Geometry: final body of the model. Coordinates: model frame, mm. A direction names the side the tool comes from. Round coordinates to 2 decimals unless told otherwise and drop trailing zeros. Loops run counter-clockwise (first coordinate to the right, second up) from the corner with the lowest first, then second, coordinate; pieces in that order, holes last. Notation, with made-up numbers: (-10.75, -11.75) - (47.25, -11.75) arc R25 cw to (47.25, 23.25) - close; hole circle Ø2 at (53.5, -14.5). An arc over 180 degrees is marked (long way). Answer as a JSON object with one key per item and string values. Group by question number.
Item 1: Section A-A (z = 0.25). Return the cut outline in (x, y).
Item 2: First-contact query: pin 1 (1 mm diameter, centred on x = -0.5, y = 4.5, fed in from -Z); pin 2 (1.5 mm diameter, centred on x = 1.5, y = 8.5, fed in from +Z); pin 3 (5 mm diameter, centred on y = 8, z = 1, fed in from +X). Flat tips, straight axial feed; report the tip coordinate or a pass-through.
Item 3: Reachability of faces 4 (the face through (0, 12, -3)), 5 (the face through (6.554, 6, 0)), 6 (the face through (0.103, 6.085, -5.885)), 7 (the face through (-2.1, 10.8, 5.8)), 8 (the face through (0, 12, 3)) from +Z, -Z, +X, -X, +Y, -Y: full face, straight path, thin tool, end or side. Return the list, or none.
Item 4: Line query: line 1 (Y direction, x = 6.5, z = 4.75); line 2 (X direction, y = -0.5, z = -4.75); line 3 (X direction, y = 3, z = -0.75). Output: solid intervals per line, ascending.
Item 5: Draft query along Y for faces 1 (the face through (-7.1, 12, 0)), 2 (the face through (0, 0, 0)), 3 (the face through (-2.1, 1.5, 5.8)). Return one class per face: released by +Y, released by -Y, zero draft, split by the parting line, or undercut.
Item 6: Section C-C (y = 7.25). Return the cut outline in (x, z), plus the area to 3 significant figures.
Item 7: Section B-B (x = -3.5). Return the cut outline in (y, z).
Item 8: Section D-D (x = -6). Return the cut outline in (y, z).
```python
from build123d import *

# Parameters (mm, degrees)
SKETCH_1_W           = 14.2
SKETCH_1_H           = 12.2
EXTRUDE_1_DEPTH      = 12.8
SKETCH_2_OUTSIDE_W   = 20.736
SKETCH_2_OUTSIDE_H   = 18.736
SKETCH_2_OUTSIDE_W_2 = 19.736348523
SKETCH_2_OUTSIDE_H_2 = 6
CUT_EXTRUDE_1_DEPTH  = 1.5
SKETCH_3_OUTSIDE_W   = 20.736
SKETCH_3_OUTSIDE_H   = 18.736
CUT_EXTRUDE_2_DEPTH  = 9.3
SKETCH_4_R           = 0.375
EXTRUDE_2_DEPTH      = 4.5


with BuildPart() as part:
    # 草图1 → 凸台-拉伸1 (new body)
    with BuildSketch(Plane(origin=(0, 0, 0), x_dir=(1, 0, 0), z_dir=(0, 1, 0))):
        Rectangle(SKETCH_1_W, SKETCH_1_H)
    extrude(amount=EXTRUDE_1_DEPTH)

    # 草图2 outside → 切除-拉伸1 (cut)
    with BuildSketch(Plane(origin=(0, 12.8, 0), x_dir=(1, 0, 0), z_dir=(0, 1, 0))):
        Rectangle(SKETCH_2_OUTSIDE_W, SKETCH_2_OUTSIDE_H)
        with Locations((-0.320715663, 0)):
            Rectangle(SKETCH_2_OUTSIDE_W_2, SKETCH_2_OUTSIDE_H_2, mode=Mode.SUBTRACT)
    extrude(amount=-CUT_EXTRUDE_1_DEPTH, mode=Mode.SUBTRACT)

    # 草图3 outside → 切除-拉伸2 (cut)
    with BuildSketch(Plane(origin=(0, 1.5, 0), x_dir=(1, 0, 0), z_dir=(0, 1, 0))):
        Rectangle(SKETCH_3_OUTSIDE_W, SKETCH_3_OUTSIDE_H)
        with BuildLine():
            Line((-6.554198564, 3), (-6.554198564, -3))
            ThreePointArc((-6.554198564, -3), (0, -5.885804343), (6.554198564, -3))
            Line((6.554198564, -3), (6.554198564, 3))
            ThreePointArc((6.554198564, 3), (0, 5.885804343), (-6.554198564, 3))
        make_face(mode=Mode.SUBTRACT)
    extrude(amount=CUT_EXTRUDE_2_DEPTH, mode=Mode.SUBTRACT)

    # 草图4 → 凸台-拉伸2 (add)
    with BuildSketch(Plane.XZ):
        with Locations(Location((-5.085, 4.445, 0), (0, 0, 90))):
            Circle(SKETCH_4_R)
        with Locations(Location((-2.545, 4.445, 0), (0, 0, 90))):
            Circle(SKETCH_4_R)
        with Locations(Location((2.545, 4.445, 0), (0, 0, 90))):
            Circle(SKETCH_4_R)
        with Locations(Location((5.085, 4.445, 0), (0, 0, 90))):
            Circle(SKETCH_4_R)
        with Locations(Location((5.085, -4.445, 0), (0, 0, 90))):
            Circle(SKETCH_4_R)
        with Locations(Location((2.545, -4.445, 0), (0, 0, 90))):
            Circle(SKETCH_4_R)
        with Locations(Location((-2.545, -4.445, 0), (0, 0, 90))):
            Circle(SKETCH_4_R)
        with Locations(Location((-5.085, -4.445, 0), (0, 0, 90))):
            Circle(SKETCH_4_R)
    extrude(amount=EXTRUDE_2_DEPTH)


solid = part.part
```
Values:
{
 "1": {"outline": "(-7.1, 0) - (7.1, 0) - (7.1, 1.5) - (6.55, 1.5) - (6.55, 10.8) - (7.1, 10.8) - (7.1, 12.8) - (-7.1, 12.8) - (-7.1, 10.8) - (-6.55, 10.8) - (-6.55, 1.5) - (-7.1, 1.5) - close"},
 "2": {"pin 1": "stops at z = -5.89", "pin 2": "stops at z = 5.85", "pin 3": "stops at x = 6.55"},
 "3": {"face 4": "-Z, +X, -X, +Y", "face 5": "+Z, -Z, +X", "face 6": "-Z", "face 7": "none", "face 8": "+Z, +X, -X, +Y"},
 "4": {"line 1": "y = 0 to 1.5, 10.8 to 11.3", "line 2": "x = -5.3 to -4.87, -2.76 to -2.33, 2.33 to 2.76, 4.87 to 5.3", "line 3": "x = -6.55 to 6.55"},
 "5": {"face 1": "zero draft", "face 2": "released by -Y", "face 3": "undercut"},
 "6": {"outline": "(-6.55, -3) arc R8.89 ccw to (6.55, -3) - (6.55, 3) arc R8.89 ccw to (-6.55, 3) - close", "area": "131 mm^2"},
 "7": {"outline": "(0, -6.1) - (1.5, -6.1) - (1.5, -5.17) - (10.8, -5.17) - (10.8, -6.1) - (11.3, -6.1) - (11.3, -3) - (12.8, -3) - (12.8, 3) - (11.3, 3) - (11.3, 6.1) - (10.8, 6.1) - (10.8, 5.17) - (1.5, 5.17) - (1.5, 6.1) - (0, 6.1) - close"},
 "8": {"outline": "(0, -6.1) - (1.5, -6.1) - (1.5, -3.55) - (10.8, -3.55) - (10.8, -6.1) - (11.3, -6.1) - (11.3, -3) - (12.8, -3) - (12.8, 3) - (11.3, 3) - (11.3, 6.1) - (10.8, 6.1) - (10.8, 3.55) - (1.5, 3.55) - (1.5, 6.1) - (0, 6.1) - close"}
}
